The model under review builds one solid part; all positions refer to its coordinate system, in mm. A direction names the side the tool comes from. Round coordinates to 2 decimals unless told otherwise and drop trailing zeros. Loops run counter-clockwise (first coordinate to the right, second up) from the corner with the lowest first, then second, coordinate; pieces in that order, holes last. Notation, with made-up numbers: M 1.25,66 L 45.25,66 A26 cw 45.25,92 Z; hole C -33,-34 d8. An arc over 180 degrees is marked long. Answer as a JSON object with one key per item and string values. Group by question number.
Item 1: Consider section D-D (x = 5). Give the boundary of the cut face in (y, z), and give its area (3 significant figures).
Item 2: Insertion check: P1, Ø17.5, axis at x = 12.5, z = -23.5, coming from the +Y side; P2, Ø6, axis at y = 132, z = -21.5, coming from the -X side. Each pin has a flat end and moves straight along its axis. Give the tip position at first contact, or say it passes through.
Item 3: To check wall thickness, follow line 1 (Y direction, x = 3, z = -33); line 2 (X direction, y = 169.5, z = -30); line 3 (Y direction, x = 23, z = -11.5). State the ranges of each line that lie inside material, in increasing order.
Item 4: Consider section C-C (y = 27.5). Give the boundary of the cut face in (x, z) (3 decimals), and give its area (3 significant figures).
Item 5: Consider section A-A (z = -6.5). Give the boundary of the cut face in (x, y) (3 decimals), and give its area (3 significant figures).
Item 6: Consider section B-B (x = 51.5). Give the boundary of the cut face in (y, z) (3 decimals), and give its area (3 significant figures).
Item 7: Tool access review of faces 1 (the face through (11, 0, -19)), 2 (the face through (11, 38.1, -19)): name each direction out of +Z, -Z, +X, -X, +Y, -Y from which nothing blocks a thin tool from reaching the whole face with its end or side.
```python
from build123d import *

# Parameters (mm, degrees)
SKETCH1_W   = 38.1
SKETCH1_H   = 38.1
SKETCH1_W_2 = 31.75
SKETCH1_H_2 = 31.75
SKETCH3_W   = 31.75
SKETCH3_H   = 31.75


with BuildPart() as part:
    # Sweep1: sweep along a path in Sketch2
    with BuildLine(Plane.XY) as sweep1_path:
        Line((40.95, 179.05), (40.95, 38.1))
        ThreePointArc((40.95, 38.1), (35.370384182, 24.629615818), (21.9, 19.05))
        Line((21.9, 19.05), (0, 19.05))
    # Sketch1 → Sweep1 (sweep)
    with BuildSketch(Plane(origin=(0, 0, 0), x_dir=(0, 0, -1), z_dir=(1, 0, 0))):
        with Locations((19.05, 19.05)):
            Rectangle(SKETCH1_W, SKETCH1_H)
        with Locations((19.05, 19.05)):
            Rectangle(SKETCH1_W_2, SKETCH1_H_2, mode=Mode.SUBTRACT)
    sweep(path=sweep1_path.line)

    # Sweep2: sweep along a path in Sketch2<2>
    with BuildLine(Plane.XY) as sweep2_path:
        Line((40.95, 179.05), (40.95, 38.1))
        ThreePointArc((40.95, 38.1), (35.370384182, 24.629615818), (21.9, 19.05))
        Line((21.9, 19.05), (0, 19.05))
    # Sketch3 → Sweep2 (sweep)
    with BuildSketch(Plane(origin=(0, 179.05, 0), x_dir=(1, 0, 0), z_dir=(0, 1, 0))):
        with Locations((40.95, 19.05)):
            Rectangle(SKETCH3_W, SKETCH3_H)
    sweep(path=sweep2_path.line)


solid = part.part
```
Geometry results:
{
 "1": {"outline": "M 0,-38.1 L 38.1,-38.1 L 38.1,0 L 0,0 Z", "area": "1,450 mm^2"},
 "2": {"P1": "stops at y = 38.1", "P2": "stops at x = 21.9"},
 "3": {"line 1": "y = 0 to 38.1", "line 2": "x = 21.9 to 60", "line 3": "y = 0.02 to 179.05"},
 "4": {"outline": "M 0,-38.1 L 58.496,-38.1 L 58.496,0 L 0,0 Z", "area": "2,230 mm^2"},
 "5": {"outline": "M 0,0 L 21.9,0 A38.1 ccw 60,38.1 L 60,179.05 L 21.9,179.05 L 21.9,38.1 L 0,38.1 Z", "area": "7,340 mm^2"},
 "6": {"outline": "M 14.111,-38.1 L 179.05,-38.1 L 179.05,0 L 14.111,0 Z", "area": "6,280 mm^2"},
 "7": {"face 1": "+Z, -Z, +X, -X, -Y", "face 2": "+Z, -Z, -X, +Y"}
}
